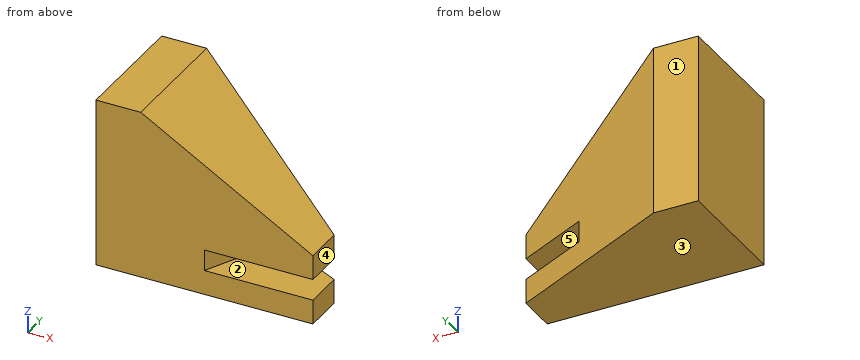
Autodesk Inventor part; units mm, degrees
ref_plane "YZ Plane" through (0, 0, 0) normal (1, 0, 0) x (0, 1, 0)
ref_plane "XZ Plane" through (0, 0, 0) normal (0, 1, 0) x (-1, 0, 0)
ref_plane "XY Plane" through (0, 0, 0) normal (0, 0, 1) x (1, 0, 0)
sketch "Sketch1" plane through (0, 0, 0) normal (0, 0, 1) x (1, 0, 0)
  line L0 (0, 0) -> (32.4623, 0)
  line L1 (32.4623, 0) -> (32.4623, 18.6079)
  line L2 (32.4623, 18.6079) -> (0, 18.6079)
  line L3 (0, 18.6079) -> (0, 0)
extrude "Extrusion1" add sketch "Sketch1" along normal blind 25.4
sketch "Sketch2" plane through (0, 0, 25.4) normal (0, 0, 1) x (1, 0, 0)
  line L0 (32.4623, 0) -> (32.4623, 18.6079)
  line L1 (32.4623, 18.6079) -> (0, 18.6079)
  line L2 (6.7125, 18.6079) -> (32.4623, 6.0135)
extrude "Extrusion2" cut sketch "Sketch2" against normal through all
sketch "Sketch4" plane through (0, 18.6079, 25.4) normal (0, 1, 0) x (1, 0, 0)
  line L0 (0, 25.4) -> (0, 0)
  line L1 (6.7125, 25.4) -> (32.4623, 25.4)
  line L2 (6.7125, 0) -> (6.7125, 25.4)
  line L3 (32.4623, 0) -> (6.7125, 0)
  line L4 (32.4623, 25.4) -> (32.4623, 0)
  line L5 (6.7125, 0) -> (32.4623, 14.8667)
  dimension "d6" = 30
extrude "Extrusion4" cut sketch "Sketch4" against normal through all contours L5 L4 L3
ref_plane "Work Plane1" through (32.4623, 6.0135, 5.2667) normal (0, 0, 1) x (1, 0, 0)
sketch "Sketch5" plane through (32.4623, 6.0135, 5.2667) normal (0, 0, 1) x (1, 0, 0)
  line L0 (-32.4623, -6.0135) -> (-32.4623, 12.5943)
  line L1 (-32.4623, 12.5943) -> (-25.7498, 12.5943)
  line L2 (-25.7498, 12.5943) -> (0, 0)
  line L3 (0, 0) -> (0, -6.0135)
  line L4 (0, -6.0135) -> (-32.4623, -6.0135)
  line L5 (-16.2312, -6.0135) -> (-10.7244, 5.2453)
extrude "Extrusion5" cut sketch "Sketch5" along normal mid plane 3.175 contours L5 L2 L3 L4
properties part number "Importing AutoCAD Geometry"
Design review of the part built by this model. Coordinates are the model's own, in mm. Face numbers are marked on the shaded views. A direction names the side the tool comes from. Coordinates: 2 decimals unless noted, no trailing zeros. Write each loop counter-clockwise with the first axis right and the second up, starting at its lowest first coordinate (ties: lowest second). Pieces come first, ordered by that corner, then holes. Notation, with made-up numbers: (65, 65.5) - (86, 65.5) arc R22 ccw to (86, 73.5) - close; hole circle Ø1 at (-33, 15.25). An arc over 180 degrees is marked (long way). One line per item, written item: value.
1) For the marked faces 1 and 2, list the 3-axis set-ups (+Z, -Z, +X, -X, +Y, -Y) from which the entire face can be reached by the end or side of a thin tool; tool diameter is ignored.
Answer sheet:
face 1: +Z, -Z, +X, -X, +Y
face 2: +X, -Y
2) Add section C-C (y = 8). State the section outline as (x, z) points.
Answer sheet:
outline: (0, 0) - (28.4, 0) - (28.4, 3.68) - (20.14, 3.68) - (20.14, 6.85) - (28.4, 6.85) - (28.4, 12.88) - (6.71, 25.4) - (0, 25.4) - close
3) To check wall thickness, follow probe 1 along X at (y, z) = (11.25, 18.25); probe 2 along Z at (x, y) = (28, 5.25); probe 3 along X at (y, z) = (9.75, 7). State the ranges of each line that lie inside material, in increasing order.
Answer sheet:
probe 1: x = 0 to 19.1
probe 2: z = 0 to 3.68, 6.85 to 13.11
probe 3: x = 0 to 24.82
4) Add section D-D (x = 19). State the section outline as (y, z) points.
Answer sheet:
outline: (0, 0) - (12.6, 0) - (12.6, 18.31) - (0, 18.31) - (0, 6.85) - (5.66, 6.85) - (5.66, 3.68) - (0, 3.68) - close
5) Insertion check: pin 1 (5 mm diameter, centred on x = 28.5, y = 11, fed in from +Z); pin 2 (2 mm diameter, centred on x = 24, y = 7, fed in from +Z); pin 3 (1.5 mm diameter, centred on y = 14, z = 13, fed in from +X); pin 4 (3 mm diameter, centred on x = 18.5, z = 7, fed in from +Y). Each pin has a flat end and moves straight along its axis. Give the tip position at first contact, or say it passes through.
Answer sheet:
pin 1: passes through
pin 2: stops at z = 16
pin 3: stops at x = 17.67
pin 4: stops at y = 13.58
6) Add section A-A (x = 28). State the section outline as (y, z) points.
Answer sheet:
outline: (0, 0) - (8.2, 0) - (8.2, 3.68) - (0, 3.68) - close; (0, 6.85) - (8.2, 6.85) - (8.2, 13.11) - (0, 13.11) - close
7) Mouldability with a two-part tool opening along Z and no side actions: class the marked faces 3, 4 and 5 as +Z half, -Z half, draft (parallel to the pull), parting line (faces both ways), or undercut.
Answer sheet:
face 3: -Z half
face 4: draft
face 5: undercut
8) Add section B-B (z = 2.75). State the section outline as (x, y) points.
Answer sheet:
outline: (0, 0) - (32.46, 0) - (32.46, 6.01) - (6.71, 18.61) - (0, 18.61) - close
